Here's how the part is built. I have some questions about the finished solid (model axes, mm). Give positions to 0.01 mm unless a question says otherwise; leave off trailing zeros. Write each loop counter-clockwise with the first axis right and the second up, starting at its lowest first coordinate (ties: lowest second). Pieces come first, ordered by that corner, then holes. Notation, with made-up numbers: (87.25, 49.5) -> (126.25, 49.5) arc R28 cw to (126.25, 72.5) -> close; hole circle Ø7 at (64, 57). An arc over 180 degrees is marked (long way). Return JSON: item names as keys, results as strings.
from build123d import *

# Parameters (mm, degrees)
SKETCH1_R                 = 1.905
BOSS_EXTRUDE1_DEPTH       = 20.32
F_4_40_TAPPED_HOLE1_D     = 2.2606
F_4_40_TAPPED_HOLE1_DEPTH = 7.62
F_4_40_TAPPED_HOLE1_TIP   = 0.679152758
CUT_EXTRUDE1_DEPTH        = 21.497815737
CUT_EXTRUDE1_DEPTH_BACK   = 21.497815737
SKETCH4_R                 = 1.27


with BuildPart() as part:
    # Sketch1 → Boss-Extrude1 (new body)
    with BuildSketch(Plane(origin=(0, 0, 0), x_dir=(1, 0, 0), z_dir=(0, 1, 0))):
        with Locations(Location((0, 0, 0), (0, 0, 270))):
            Circle(SKETCH1_R)
    extrude(amount=-BOSS_EXTRUDE1_DEPTH)

    # #4-40 Tapped Hole1
    with Locations(Plane(origin=(0, 0, 0), x_dir=(1, 0, 0), z_dir=(0, 1, 0))):
        with Locations((0, 0)):
            Hole(F_4_40_TAPPED_HOLE1_D / 2, depth=F_4_40_TAPPED_HOLE1_DEPTH)
            with Locations((0, 0, -(F_4_40_TAPPED_HOLE1_DEPTH + F_4_40_TAPPED_HOLE1_TIP / 2))):  # 118° drill point
                Cone(0, F_4_40_TAPPED_HOLE1_D / 2, F_4_40_TAPPED_HOLE1_TIP, mode=Mode.SUBTRACT)

    # Sketch4 → Cut-Extrude1 (cut, two sides: drawn at the far end of the back side and taken through both)
    with BuildSketch(Plane.XY.offset(-CUT_EXTRUDE1_DEPTH_BACK)):
        with Locations(Location((0, -17.018, 0), (0, 0, 90.000000002))):
            Circle(SKETCH4_R)
    extrude(amount=CUT_EXTRUDE1_DEPTH + CUT_EXTRUDE1_DEPTH_BACK, mode=Mode.SUBTRACT)


solid = part.part
1. Suppose I cut it at A-A, the plane y = -2.25. List the corners of the cut face in (x, z) for me (3 decimals).
Taken from the geometry:
{"outline": "circle Ø3.81 at (0, 0); hole circle Ø2.261 at (0, 0)"}
2. If we mould it in two halves opening along X, with no side actions, what happens to faces 1 (the face through (1.89, -10.02, -0.25)), 2 (the face through (0.245, -3.863, 1.103)), 3 (the face through (0, -20.32, 0))? For each: released by +X, released by -X, zero draft, split by the parting line, or undercut.
Taken from the geometry:
{"face 1": "split by the parting line", "face 2": "undercut", "face 3": "zero draft"}
3. Suppose I cut it at B-B, the plane y = -17.75. List the corners of the cut face in (x, z) for me (3 decimals).
Taken from the geometry:
{"outline": "(-1.038, -1.597) -> (-1.038, 1.597) arc R1.905 ccw to start; (1.038, -1.597) arc R1.905 ccw to (1.038, 1.597) -> close"}
4. For pin 1 Ø1 at (x, z) = (0, 0.5) entering from +Y, with a flat end and sliding along its axis, tell me the tip position at first contact or that it passes through.
Taken from the geometry:
{"pin 1": "stops at y = -7.7"}
5. Suppose I cut it at C-C, the plane y = -13.5. List the corners of the cut face in (x, z) for me (3 decimals), and give its area (3 significant figures).
Taken from the geometry:
{"outline": "circle Ø3.81 at (0, 0)", "area": "11.4 mm²"}
6. If I drill on line 1 (Z direction, x = 0, y = -3) (3 decimals); line 2 (X direction, y = -3, z = 0.95); line 3 (X direction, y = -3.25, z = -0.55), over which ranges is the centre line in solid material (lowest first)? Write a range as [from, to].
Taken from the geometry:
{"line 1": "z = [-1.905, -1.13], [1.13, 1.905]", "line 2": "x = [-1.65, -0.61], [0.61, 1.65]", "line 3": "x = [-1.82, -0.99], [0.99, 1.82]"}
